Geometry: see drawing. Coordinates: mm, zero at the bounding-box minimum. Round coordinates to 2 decimals unless told otherwise and drop trailing zeros. Write each loop counter-clockwise with the first axis right and the second up, starting at its lowest first coordinate (ties: lowest second). Pieces come first, ordered by that corner, then holes. Notation, with made-up numbers: (11.25, 73) -> (68.25, 73) arc R24 ccw to (68.25, 89) -> close; hole circle Ø7 at (-6, -4.5). An arc over 180 degrees is marked (long way). Write item = value, one per line.
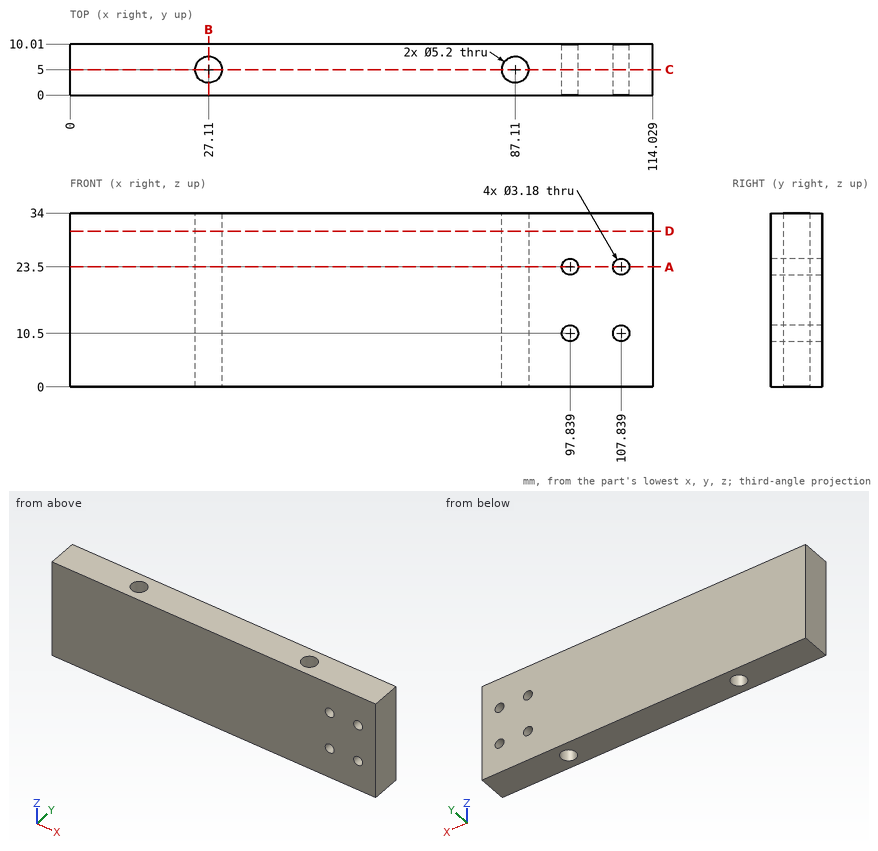
1) Cut plane C-C (y = 5). Return the cut outline in (x, z), and give its area (3 significant figures).
Solutions:
outline = (0, 0) -> (24.51, 0) -> (24.51, 34) -> (0, 34) -> close; (29.71, 0) -> (84.51, 0) -> (84.51, 34) -> (29.71, 34) -> close; (89.71, 0) -> (114.03, 0) -> (114.03, 34) -> (89.71, 34) -> close; hole circle Ø3.18 at (97.84, 10.5); hole circle Ø3.18 at (97.84, 23.5); hole circle Ø3.18 at (107.84, 10.5); hole circle Ø3.18 at (107.84, 23.5)
area = 3,490 mm^2
2) Cut plane A-A (z = 23.5). Return the cut outline in (x, y).
Solutions:
outline = (0, 0) -> (96.25, 0) -> (96.25, 10.01) -> (0, 10.01) -> close; (99.43, 0) -> (106.25, 0) -> (106.25, 10.01) -> (99.43, 10.01) -> close; (109.43, 0) -> (114.03, 0) -> (114.03, 10.01) -> (109.43, 10.01) -> close; hole circle Ø5.2 at (27.11, 5); hole circle Ø5.2 at (87.11, 5)
3) Cut plane D-D (z = 30.5). Return the cut outline in (x, y).
Solutions:
outline = (0, 0) -> (114.03, 0) -> (114.03, 10.01) -> (0, 10.01) -> close; hole circle Ø5.2 at (27.11, 5); hole circle Ø5.2 at (87.11, 5)
4) Cut plane B-B (x = 27.11). Return the cut outline in (y, z).
Solutions:
outline = (0, 0) -> (2.4, 0) -> (2.4, 34) -> (0, 34) -> close; (7.6, 0) -> (10.01, 0) -> (10.01, 34) -> (7.6, 34) -> close
5) Line query: L1, parallel to X at y = 5.25, z = 26; L2, parallel to Y at x = 87, z = 27; L3, parallel to X at y = 2.75, z = 3.5. Output: solid intervals per line, ascending. Write a range as from..to.
Solutions:
L1 = 0..24.52, 29.7..84.52, 89.7..114.03
L2 = 0..2.4, 7.6..10.01
L3 = 0..25.81, 28.41..85.81, 88.41..114.03
